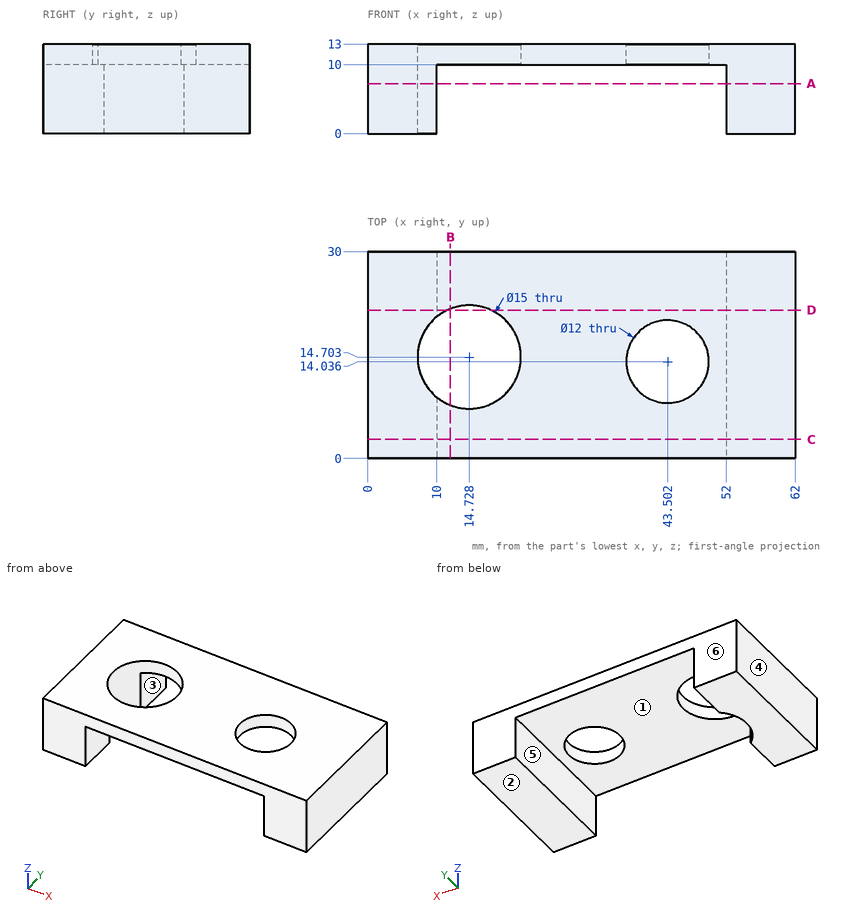
Design review of the part shown in the three views and the two pictorial views. Dimensions are in mm from the part's minimum x, y and z. A direction names the side the tool comes from. Give positions to 0.01 mm unless a question says otherwise; leave off trailing zeros. Write each loop counter-clockwise with the first axis right and the second up, starting at its lowest first coordinate (ties: lowest second). Pieces come first, ordered by that corner, then holes. Notation, with made-up numbers: M 62.25,19.25 L 109.25,19.25 A26 cw 109.25,48.25 Z; hole C -19.75,-37.75 d4. An arc over 180 degrees is marked long. One line per question, with ' | ' between items. Start each with the question number.
Item 1: Draft analysis for pull direction X (two halves, no side actions). For the marked faces 3, 4, 5 and 6, state which applies: released by +X, released by -X, zero draft, split by the parting line, or undercut.
Item 2: We need section B-B on x = 12. Write out the cut boundary in (y, z).
Item 3: For pin 1 (13.5 mm diameter, centred on x = 14.73, y = 14.7, fed in from -Z); pin 2 (1 mm diameter, centred on x = 36.5, y = 20, fed in from -Z), all flat-tipped, find the tip position at first contact; note any pin that passes through.
Item 4: We need section A-A on z = 7.25. Write out the cut boundary in (x, y) (1 decimal).
Item 5: For the marked faces 1 and 2, list the 3-axis set-ups (+Z, -Z, +X, -X, +Y, -Y) from which the entire face can be reached by the end or side of a thin tool; tool diameter is ignored.
Item 6: We need section D-D on y = 21.5. Write out the cut boundary in (x, z).
Item 7: We need section C-C on y = 2.75. Write out the cut boundary in (x, z), plus the area to 3 significant figures.
Item 8: Wall thickness on line 1 (X direction, y = 22.5, z = 6.5); line 2 (Z direction, x = 42, y = 23.75); line 3 (Y direction, x = 38, z = 10.5) (1 decimal): over which ranges is each line inside the solid? List them lowest first. Write a range as from..to.
Results found:
1) face 3: undercut | face 4: released by -X | face 5: undercut | face 6: zero draft
2) outline: M 0,10 L 7.72,10 L 7.72,13 L 0,13 Z; M 21.69,10 L 30,10 L 30,13 L 21.69,13 Z
3) pin 1: passes through | pin 2: stops at z = 10
4) outline: M 0,0 L 10,0 L 10,8.9 A7.5 cw 10,20.5 L 10,30 L 0,30 Z; M 52,0 L 62,0 L 62,30 L 52,30 Z
5) face 1: -Z, +Y, -Y | face 2: -Z, +X, -X, +Y, -Y
6) outline: M 0,0 L 10,0 L 10,10 L 11.56,10 L 11.56,13 L 0,13 Z; M 17.9,10 L 52,10 L 52,0 L 62,0 L 62,13 L 17.9,13 Z
7) outline: M 0,0 L 10,0 L 10,10 L 52,10 L 52,0 L 62,0 L 62,13 L 0,13 Z | area: 386 mm2
8) line 1: x = 0..10, 52..62 | line 2: z = 10..13 | line 3: y = 0..11.6, 16.4..30
